The drawing under review shows one solid part. Ordinate dimensions are in mm from its lowest x, y, z. A direction names the side the tool comes from. Coordinates: 2 decimals unless noted, no trailing zeros. Order: outer loops, then holes, each group sorted by start corner. A loop starts at its lowest first (then second) coordinate and runs counter-clockwise, first axis right, second up.
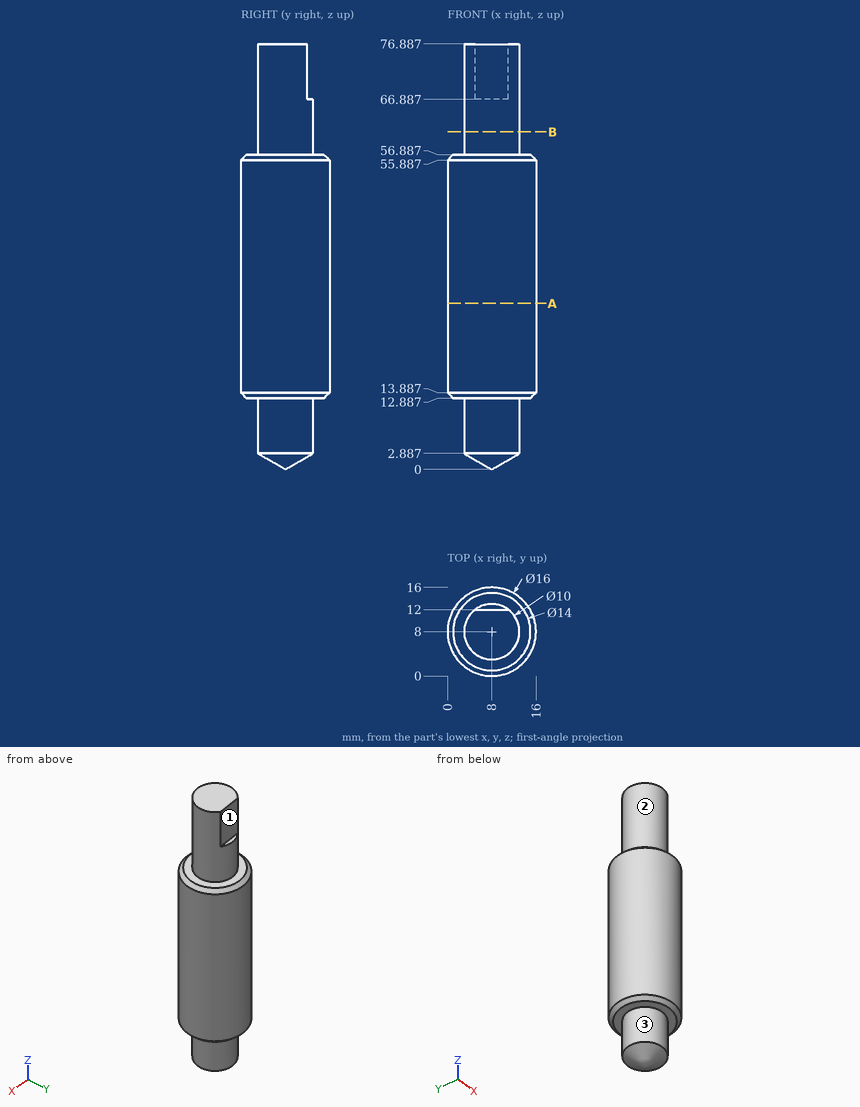
(1) Machinability: for the marked faces 1, 2 and 3, which of the approach directions +Z, -Z, +X, -X, +Y, -Y give a long, thin tool a straight path to every point of the face, cutting with its end or side? Answer none if there is none.
A:
face 1: +Z, +X, -X, +Y
face 2: +Z
face 3: -Z
(2) For pin 1 Ø6 at (x, y) = (14, 3.5) entering from -Z; pin 2 Ø1.5 at (x, z) = (7, 51.5) entering from -Y; pin 3 Ø5 at (y, z) = (14, 38.5) entering from +X, all flat-tipped, find the tip position at first contact; note any pin that passes through.
A:
pin 1: stops at z = 2.6
pin 2: stops at y = 0
pin 3: stops at x = 15.19
(3) Wall thickness on probe 1 along Z at (x, y) = (6.5, 1.75); probe 2 along Y at (x, z) = (8.25, 18.5); probe 3 along X at (y, z) = (4, 61): over which ranges is each line inside the solid? List them lowest first.
A:
probe 1: z = 12.89 to 56.89
probe 2: y = 0 to 16
probe 3: x = 5 to 11
(4) We need section B-B, the plane z = 61. Write out the cut boundary in (x, y).
A:
outline: circle Ø10 at (8, 8)
(5) We need section A-A, the plane z = 30. Write out the cut boundary in (x, y).
A:
outline: circle Ø16 at (8, 8)
